Geometry: final body of the model. Coordinates: model frame, mm. Face numbers are marked on the shaded views. A direction names the side the tool comes from. Give positions to 0.01 mm unless a question says otherwise; leave off trailing zeros. Write each loop counter-clockwise with the first axis right and the second up, starting at its lowest first coordinate (ties: lowest second). Pieces come first, ordered by that corner, then holes. Notation, with made-up numbers: (26.5, -23) -> (62.5, -23) arc R12 ccw to (62.5, -19) -> close; hole circle Ø5 at (66.25, -5). An arc over 180 degrees is marked (long way). Answer in a Markdown table with one row per item. Add a question column.
from build123d import *

# Parameters (mm, degrees)
SKETCH_1_W          = 27.4
SKETCH_1_H          = 6.7
EXTRUDE_1_DEPTH     = 1.4
SKETCH_2_W          = 3
SKETCH_2_H          = 8.022879097
EXTRUDE_2_DEPTH     = 1.78
SKETCH_3_W          = 33.4
SKETCH_3_H          = 8.022879097
EXTRUDE_6_DEPTH     = 0.58
SKETCH_4_R          = 1.2
CUT_EXTRUDE_1_DEPTH = 1
SKETCH_6_W          = 33.4
SKETCH_6_H          = 8.022879097
CUT_EXTRUDE_3_DEPTH = 0.1
SKETCH_7_W          = 3.66
SKETCH_7_H          = 8.022879097
EXTRUDE_7_DEPTH     = 4
SKETCH_8_R          = 2.5
CUT_EXTRUDE_4_DEPTH = 2.5
SKETCH_9_R          = 1
CUT_EXTRUDE_5_DEPTH = 5
SKETCH_10_W         = 3.66
SKETCH_10_H         = 8.022879097
EXTRUDE_8_DEPTH     = 4
SKETCH_11_R         = 2.5
CUT_EXTRUDE_6_DEPTH = 2.5
SKETCH_12_R         = 1
CUT_EXTRUDE_7_DEPTH = 2.5


with BuildPart() as part:
    # 스케치1 → 보스-돌출1 (new body)
    with BuildSketch(Plane.XY):
        Polygon((-16.7, -0.330719774), (16.7, -0.330719774), (16.7, 0.330719774), (16.7, 7.030719774), (16.7, 7.692159323), (-16.7, 7.692159323), (-16.7, 7.030719774), (-16.7, 0.330719774), align=None)
        with Locations((0, 3.680719774)):
            Rectangle(SKETCH_1_W, SKETCH_1_H, mode=Mode.SUBTRACT)
    extrude(amount=EXTRUDE_1_DEPTH)

    # 스케치2 → 보스-돌출2 (add)
    with BuildSketch(Plane.XY.offset(1.4)):
        with Locations((-15.2, 3.680719774)):
            Rectangle(SKETCH_2_W, SKETCH_2_H)
        with Locations((15.2, 3.680719774)):
            Rectangle(SKETCH_2_W, SKETCH_2_H)
    extrude(amount=EXTRUDE_2_DEPTH)

    # 스케치3 → 보스-돌출6 (add)
    with BuildSketch(Plane(origin=(0, 0, 0), x_dir=(-1, 0, 0), z_dir=(0, 0, -1))):
        with Locations((0, 3.680719774)):
            Rectangle(SKETCH_3_W, SKETCH_3_H)
    extrude(amount=EXTRUDE_6_DEPTH)

    # 스케치4 → 컷-돌출1 (cut)
    with BuildSketch(Plane(origin=(0, 0, -0.58), x_dir=(-1, 0, 0), z_dir=(0, 0, -1))):
        with Locations((-9.9, 3.680719774)):
            Circle(SKETCH_4_R)
        with Locations((-3.3, 3.680719774)):
            Circle(SKETCH_4_R)
        with Locations((3.3, 3.680719774)):
            Circle(SKETCH_4_R)
        with Locations((9.9, 3.680719774)):
            Circle(SKETCH_4_R)
    extrude(amount=-CUT_EXTRUDE_1_DEPTH, mode=Mode.SUBTRACT)

    # 스케치6 → 컷-돌출3 (cut)
    with BuildSketch(Plane(origin=(0, 0, -0.58), x_dir=(-1, 0, 0), z_dir=(0, 0, -1))):
        with Locations((0, 3.680719774)):
            Rectangle(SKETCH_6_W, SKETCH_6_H)
    extrude(amount=-CUT_EXTRUDE_3_DEPTH, mode=Mode.SUBTRACT)

    # 스케치7 → 보스-돌출7 (add)
    with BuildSketch(Plane.ZY.offset(16.7)):
        with Locations((1.35, 3.680719774)):
            Rectangle(SKETCH_7_W, SKETCH_7_H)
    extrude(amount=EXTRUDE_7_DEPTH)

    # 스케치8 → 컷-돌출4 (cut)
    with BuildSketch(Plane(origin=(0, 0, -0.48), x_dir=(-1, 0, 0), z_dir=(0, 0, -1))):
        with Locations((17.2, 3.680719774)):
            Circle(SKETCH_8_R)
    extrude(amount=-CUT_EXTRUDE_4_DEPTH, mode=Mode.SUBTRACT)

    # 스케치9 → 컷-돌출5 (cut)
    with BuildSketch(Plane(origin=(0, 0, 2.02), x_dir=(-1, 0, 0), z_dir=(0, 0, -1))):
        with Locations((17.2, 3.680719774)):
            Circle(SKETCH_9_R)
    extrude(amount=-CUT_EXTRUDE_5_DEPTH, mode=Mode.SUBTRACT)

    # 스케치10 → 보스-돌출8 (add)
    with BuildSketch(Plane(origin=(16.7, 0, 0), x_dir=(0, 0, -1), z_dir=(1, 0, 0))):
        with Locations((-1.35, 3.680719774)):
            Rectangle(SKETCH_10_W, SKETCH_10_H)
    extrude(amount=EXTRUDE_8_DEPTH)

    # 스케치11 → 컷-돌출6 (cut)
    with BuildSketch(Plane(origin=(0, 0, -0.48), x_dir=(-1, 0, 0), z_dir=(0, 0, -1))):
        with Locations((-17.2, 3.680719774)):
            Circle(SKETCH_11_R)
    extrude(amount=-CUT_EXTRUDE_6_DEPTH, mode=Mode.SUBTRACT)

    # 스케치12 → 컷-돌출7 (cut)
    with BuildSketch(Plane(origin=(0, 0, 2.02), x_dir=(-1, 0, 0), z_dir=(0, 0, -1))):
        with Locations((-17.2, 3.680719774)):
            Circle(SKETCH_12_R)
    extrude(amount=-CUT_EXTRUDE_7_DEPTH, mode=Mode.SUBTRACT)


solid = part.part
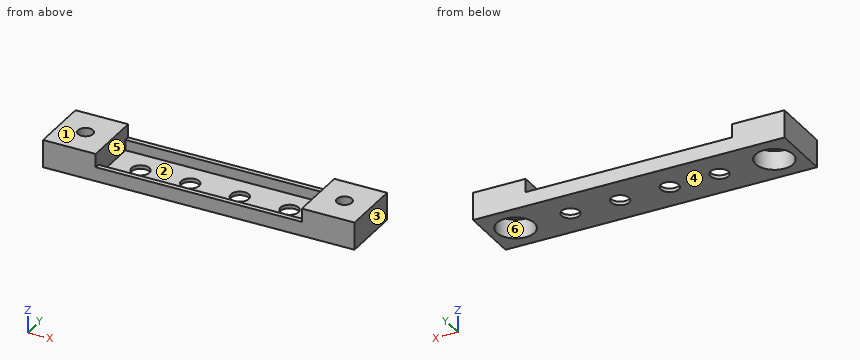
Q1. Section D-D on z = 0.4. Return loops of the section in (x, y), and give its area (3 significant figures).
Q2. Section B-B on z = 2.5. Return loops of the section in (x, y), and give its area (3 significant figures).
Q3. Line query: probe 1 along X at (y, z) = (6.25, 0.7); probe 2 along Y at (x, z) = (-9.9, -0.15); probe 3 along X at (y, z) = (4.5, 1.6). Output: solid intervals per line, ascending. Write a range as from..to.
Q4. Contact query for flat-ended pins moving along their axis: pin 1 Ø2.5 at (x, y) = (-17.2, 3.68) entering from -Z; pin 2 Ø1.6 at (x, y) = (17.2, 3.68) entering from -Z; pin 3 Ø3 at (x, y) = (-3.3, 3.68) entering from +Z. Output: stop coordinate, or through.
Q5. Pull-direction query (X, two-part tool) for the marked faces 1, 2 and 3; classes: +X half, -X half, draft (parallel to the pull), parting line (faces both ways), or undercut.
Q6. Section A-A on x = -3.3. Return loops of the section in (y, z).
Q7. Access query for the marked faces 4, 5 and 6. Directions: +Z, -Z, +X, -X, +Y, -Y. A direction counts if a zero-diameter tool reaches every point of the face in a straight line with its end or side. Return the directions, or none.
Q8. Section C-C on x = -13. Return loops of the section in (y, z).
Checks:
| question | item | result |
|---|---|---|
| 1 | outline | (-20.7, -0.33) -> (20.7, -0.33) -> (20.7, 7.69) -> (-20.7, 7.69) -> close; hole circle Ø5 at (-17.2, 3.68); hole (-13.7, 0.33) -> (13.7, 0.33) -> (13.7, 7.03) -> (-13.7, 7.03) -> close; hole circle Ø5 at (17.2, 3.68) |
| 1 | area | 109 mm^2 |
| 2 | outline | (-20.7, -0.33) -> (-13.7, -0.33) -> (-13.7, 7.69) -> (-20.7, 7.69) -> close; (13.7, -0.33) -> (20.7, -0.33) -> (20.7, 7.69) -> (13.7, 7.69) -> close; hole circle Ø2 at (-17.2, 3.68); hole circle Ø2 at (17.2, 3.68) |
| 2 | area | 106 mm^2 |
| 3 | probe 1 | -20.7..-13.7, 13.7..20.7 |
| 3 | probe 2 | -0.33..2.48, 4.88..7.69 |
| 3 | probe 3 | -20.7..-19.56, -14.84..-13.7, 13.7..14.84, 19.56..20.7 |
| 4 | pin 1 | z = 2.02 |
| 4 | pin 2 | through |
| 4 | pin 3 | z = 0 |
| 5 | face 1 | draft |
| 5 | face 2 | undercut |
| 5 | face 3 | +X half |
| 6 | outline | (-0.33, -0.48) -> (2.48, -0.48) -> (2.48, 0) -> (0.33, 0) -> (0.33, 1.4) -> (-0.33, 1.4) -> close; (4.88, -0.48) -> (7.69, -0.48) -> (7.69, 1.4) -> (7.03, 1.4) -> (7.03, 0) -> (4.88, 0) -> close |
| 7 | face 4 | -Z, +X, -X, +Y, -Y |
| 7 | face 5 | +Z |
| 7 | face 6 | -Z |
| 8 | outline | (-0.33, -0.48) -> (7.69, -0.48) -> (7.69, 1.4) -> (7.03, 1.4) -> (7.03, 0) -> (0.33, 0) -> (0.33, 1.4) -> (-0.33, 1.4) -> close |
